Autodesk Inventor part; units mm, degrees
ref_plane "YZ Plane" through (0, 0, 0) normal (1, 0, 0) x (0, 1, 0)
ref_plane "XZ Plane" through (0, 0, 0) normal (0, 1, 0) x (-1, 0, 0)
ref_plane "XY Plane" through (0, 0, 0) normal (0, 0, 1) x (1, 0, 0)
sketch "Sketch1" plane through (0, 0, 0) normal (0, 1, 0) x (-1, 0, 0)
  line L0 (0, 0) -> (0, -253.429) construction
  line L1 (5, 0) -> (5, -253.429)
  line L2 (-5, -253.429) -> (-5, 0)
  arc A0 (5, 0) -> (-5, 0) centre (0, 0) ccw
  arc A1 (-5, -253.429) -> (5, -253.429) centre (0, -253.429) ccw
  circle A2 centre (0, 0) radius 1.65
  circle A3 centre (0, -253.429) radius 1.65
  arc A4 (5, -253.429) -> (5, 0) centre (-1489.6382, -126.7145) ccw
  arc A5 (-5, -253.429) -> (-5, 0) centre (-1499.6382, -126.7145) ccw
  circle A6 centre (5.3131, -141.429) radius 1.65
  point P0 (0, -126.7145)
  dimension "d0" = 3.3
  dimension "d1" = 3.3
  dimension "d2" = 10
  dimension "d3" = 253.429
  dimension "d16" = 1500
  dimension "d17" = 1500
  dimension "d18" = 3.3
  dimension "d19" = 112
extrude "Extrusion1" add sketch "Sketch1" along normal blind 6 contours A4 L1 A6 | L1 A6 A1 A5 A0
sketch "Sketch2" plane through (0, 6, 0) normal (0, 1, 0) x (1, 0, 0)
  line L0 (-23.0122, 130.7764) -> (18.8584, 130.7764)
  line L1 (18.8584, 130.7764) -> (18.8584, -10.1345)
  line L2 (18.8584, -10.1345) -> (-23.0122, -10.1345)
  line L3 (-23.0122, -10.1345) -> (-23.0122, 130.7764)
  line L4 (-71.0561, 282.155) -> (73.8808, 282.155)
  line L5 (73.8808, 282.155) -> (73.8808, -35.6326)
  line L6 (73.8808, -35.6326) -> (-71.0561, -35.6326)
  line L7 (-71.0561, -35.6326) -> (-71.0561, 282.155)
  point P0 (0, 0)
extrude "Extrusion2" cut sketch "Sketch2" against normal blind 10 contours L0 L1 L2 L3
properties part number "Part_5_p2"
Check sheet for the modelled part. Datum: model origin and axes. Units: mm. Round coordinates to 2 decimals unless told otherwise and drop trailing zeros. Order: outer loops, then holes, each group sorted by start corner. A loop starts at its lowest first (then second) coordinate and runs counter-clockwise, first axis right, second up. Notation, with made-up numbers: M 0,9.5 L 10,9.5 A31 cw 10,45.5 Z; hole C 44,60 d4. An arc over 180 degrees is marked long. One line per item, written item: value. Start each with the question number.
1. Section check B-B on z = -179.5. Enter the section's corners in (x, y).
2. Release check for a two-part mould opening along Z. For faces 1 (the cylindrical face through (1.03, 2.96, -191.3)), 2 (the cylindrical face through (0.36, 2.96, -251.82)), 3 (the cylindrical face through (-8.97, 2.96, -191.3)) record: released by +Z, released by -Z, zero draft, split by the parting line, or undercut.
3. Gauge pin test, flat ends, axial feed: P1, Ø6, axis at x = -6, z = -169.5, coming from the -Y side; P2, Ø2.5, axis at x = 0, z = -253.429, coming from the -Y side; P3, Ø2, axis at y = 2.5, z = -149.5, coming from the +X side; P4, Ø1, axis at y = 1, z = -226, coming from the +X side. Record the tip position at first contact, or that the pin passes through.
4. Scan lines: line 1 along X through (y, z) = (1.7, -141.5); line 2 along Z through (x, y) = (-4.5, 2.75); line 3 along Z through (x, y) = (-3.5, 2.6). Record each from-to range of solid material in increasing order.
5. Section check A-A on y = 4.95. Enter the section's corners in (x, z).
Results found:
1. outline: M -9.43,0 L 0.57,0 L 0.57,6 L -9.43,6 Z
2. face 1: released by +Z
2. face 2: undercut
2. face 3: released by -Z
3. P1: y = 0
3. P2: through
3. P3: x = -0.17
3. P4: x = 2.96
4. line 1: -10.29 to -6.96, -3.66 to -0.29
4. line 2: -255.61 to -142.86, -139.99 to -130.78
4. line 3: -257 to -130.78
5. outline: M -10.36,-130.78 A1500 ccw -5,-253.43 A5 ccw 5,-253.43 A1500 cw -0.36,-130.78 Z; hole C -5.31,-141.43 d3.3; hole C 0,-253.43 d3.3
